Geometry check sheet. Reference: the model listing, model coordinates, mm. Face numbers are marked on the shaded views. A direction names the side the tool comes from. Coordinates: 2 decimals unless noted, no trailing zeros. Loops run counter-clockwise (first coordinate to the right, second up) from the corner with the lowest first, then second, coordinate; pieces in that order, holes last. Notation, with made-up numbers: M -31.75,31 L -9.75,31 A15 cw -9.75,49 Z; hole C -10.75,-15 d7. An arc over 180 degrees is marked long. Use CSV: the item, a comma, the result in double quotes.
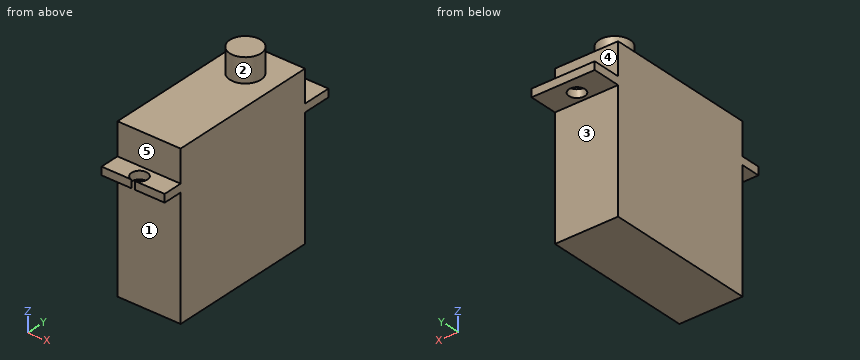
```python
from build123d import *

# Parameters (mm, degrees)
SKETCH1_W           = 20
SKETCH1_H           = 19
BOSS_EXTRUDE1_DEPTH = 7.91
SKETCH2_W           = 1
SKETCH2_H           = 25
BOSS_EXTRUDE2_DEPTH = 7.91
SKETCH3_R           = 1
CUT_EXTRUDE1_DEPTH  = 21.9
SKETCH4_R           = 1.951580775
BOSS_EXTRUDE3_DEPTH = 3


with BuildPart() as part:
    # Sketch1 → Boss-Extrude1 (new body)
    with BuildSketch(Plane(origin=(0, 0, 0), x_dir=(0, 0, -1), z_dir=(1, 0, 0))):
        with Locations((-7.960008023, 6.124197801)):
            Rectangle(SKETCH1_W, SKETCH1_H)
    extrude(amount=BOSS_EXTRUDE1_DEPTH)

    # Sketch2 → Boss-Extrude2 (add)
    with BuildSketch(Plane(origin=(7.91, 0, 0), x_dir=(0, 0, -1), z_dir=(1, 0, 0))):
        with Locations((-13.460008023, 6.694520813)):
            Rectangle(SKETCH2_W, SKETCH2_H)
    extrude(amount=-BOSS_EXTRUDE2_DEPTH)

    # Sketch3 → Cut-Extrude1 (cut)
    with BuildSketch(Plane.XY.offset(13.960008023)):
        with Locations((3.955, 17.079197801)):
            Circle(SKETCH3_R)
        with Locations((3.955, -4.830802199)):
            Circle(SKETCH3_R)
    extrude(amount=-CUT_EXTRUDE1_DEPTH, mode=Mode.SUBTRACT)

    # Sketch4 → Boss-Extrude3 (add)
    with BuildSketch(Plane.XY.offset(17.960008023)):
        with Locations((3.955, 11.333194866)):
            Circle(SKETCH4_R)
    extrude(amount=BOSS_EXTRUDE3_DEPTH)


solid = part.part
```
1. Gauge pin test, flat ends, axial feed: P1, Ø4, axis at x = 3, y = 9, coming from the +Z side; P2, Ø4, axis at x = 2, z = 7.5, coming from the +Y side; P3, Ø1.2, axis at x = 3.96, y = 17.08, coming from the +Z side; P4, Ø1.8, axis at x = 2.5, y = 18, coming from the -Z side. Record the tip position at first contact, or that the pin passes through.
The answers:
P1,"z = 20.96"
P2,"y = 15.62"
P3,"through"
P4,"z = 12.96"
2. Set-up check for the marked faces 1, 2, 3, 4 and 5: record each of +Z, -Z, +X, -X, +Y, -Y from which the full face is reachable in a straight line by a thin tool's end or side.
The answers:
face 1,"-Z, +X, -X, -Y"
face 2,"+Z"
face 3,"-Z, +X, -X, +Y"
face 4,"+Z, +X, -X, +Y"
face 5,"+Z, +X, -X, -Y"
3. Section check D-D, the plane z = 6.75. Record the cut outline in (x, y).
The answers:
outline,"M 0,-3.38 L 7.91,-3.38 L 7.91,15.62 L 0,15.62 Z"
4. Section check B-B, the plane x = 5.25. Record the cut outline in (y, z), plus the area to 3 significant figures.
The answers:
outline,"M -5.81,12.96 L -3.38,12.96 L -3.38,-2.04 L 15.62,-2.04 L 15.62,12.96 L 19.19,12.96 L 19.19,13.96 L 15.62,13.96 L 15.62,17.96 L 12.79,17.96 L 12.79,20.96 L 9.87,20.96 L 9.87,17.96 L -3.38,17.96 L -3.38,13.96 L -5.81,13.96 Z"
area,"395 mm^2"
5. Section check A-A, the plane y = 17.75. Record the cut outline in (x, z).
The answers:
outline,"M 0,12.96 L 3.21,12.96 L 3.21,13.96 L 0,13.96 Z; M 4.7,12.96 L 7.91,12.96 L 7.91,13.96 L 4.7,13.96 Z"
6. Section check C-C, the plane y = 12.5. Record the cut outline in (x, z), plus the area to 3 significant figures.
The answers:
outline,"M 0,-2.04 L 7.91,-2.04 L 7.91,17.96 L 5.52,17.96 L 5.52,20.96 L 2.39,20.96 L 2.39,17.96 L 0,17.96 Z"
area,"168 mm^2"
7. Thickness scan on line 1 (Y direction, x = 3.75, z = 10.75); line 2 (Z direction, x = 0.5, y = 9); line 3 (Z direction, x = 2.25, y = -4.5). Record the ranges inside material, lowest first. Write a range as [from, to].
The answers:
line 1,"[-3.38, 15.62]"
line 2,"[-2.04, 17.96]"
line 3,"[12.96, 13.96]"
